Source: CAD feature listing. Evaluate the final solid. Frame: model axes, mm. A direction names the side the tool comes from. Give positions to 0.01 mm unless a question says otherwise; leave off trailing zeros. Order: outer loops, then holes, each group sorted by start corner. A loop starts at its lowest first (then second) coordinate and runs counter-clockwise, first axis right, second up.
1) Access query for faces 4 (the face through (-3, 1.27, -55)), 5 (the face through (-5.3, 4.3, 0)). Directions: +Z, -Z, +X, -X, +Y, -Y. A direction counts if a zero-diameter tool reaches every point of the face in a straight line with its end or side. Return the directions, or none.
2) Section B-B, the plane z = -102. Return loops of the section in (x, y), plus the area to 3 significant figures.
3) First-contact query: P1, Ø2, axis at y = 8, z = -45.5, coming from the -X side; P2, Ø4, axis at y = 6.5, z = -90.5, coming from the -X side; P3, Ø1.7, axis at y = 3, z = -53.5, coming from the +X side. Flat tips, straight axial feed; report the tip coordinate or a pass-through.
4) Draft query along Y for faces 1 (the face through (-5.08, 3, -55)), 2 (the face through (-3, 0, -55)), 3 (the face through (-5.3, 4.3, -111.125)). Return one class per face: released by +Y, released by -Y, zero draft, split by the parting line, or undercut.
5) Section C-C, the plane y = 8.5. Return loops of the section in (x, z) (3 decimals).
6) Section A-A, the plane x = -1. Return loops of the section in (y, z) (3 decimals), plus the area to 3 significant figures.
7) Material intervals for line 1 (Y direction, x = -0.25, z = -51); line 2 (X direction, y = 4.25, z = -14.5); line 3 (Y direction, x = -3, z = -29.5), sorted ascending.
```python
from build123d import *

# Parameters (mm, degrees)
EXTRUDE_THIN1_DEPTH = 111.125
FILLET1_R           = 1.27


with BuildPart() as part:
    # Sketch1 → Extrude-Thin1 (new body)
    with BuildSketch(Plane.XY):
        with BuildLine():
            Line((0, 0), (-6.35, 0))
            Line((-6.35, 0), (-6.35, 4.7625))
            ThreePointArc((-6.35, 4.7625), (-4.490128061, 9.252628061), (0, 11.1125))
            Line((0, 11.1125), (0, 9.8425))
            ThreePointArc((0, 9.8425), (-3.592102448, 8.354602448), (-5.08, 4.7625))
            Line((-5.08, 4.7625), (-5.08, 1.27))
            Line((-5.08, 1.27), (0, 1.27))
            Line((0, 1.27), (0, 0))
        make_face()
    extrude(amount=-EXTRUDE_THIN1_DEPTH)

    # Fillet1
    fillet1_edges = [part.edges().sort_by_distance(p)[0] for p in [
        (-6.35, 0, -55.5625),
    ]]
    fillet(fillet1_edges, radius=FILLET1_R)


solid = part.part
```
From the geometry:
1. face 4: +Z, -Z, +X
1. face 5: +Z, +X, -X, +Y, -Y
2. outline: (-6.35, 1.27) arc R1.27 ccw to (-5.08, 0) - (0, 0) - (0, 1.27) - (-5.08, 1.27) - (-5.08, 4.76) arc R5.08 cw to (0, 9.84) - (0, 11.11) arc R6.35 ccw to (-6.35, 4.76) - close
2. area: 23.6 mm2
3. P1: stops at x = -5.94
3. P2: stops at x = -6.35
3. P3: stops at x = -5.08
4. face 1: undercut
4. face 2: released by -Y
4. face 3: zero draft
5. outline: (-5.134, -111.125) - (-3.441, -111.125) - (-3.441, 0) - (-5.134, 0) - close
6. outline: (0, -111.125) - (1.27, -111.125) - (1.27, 0) - (0, 0) - close; (9.743, -111.125) - (11.033, -111.125) - (11.033, 0) - (9.743, 0) - close
6. area: 284 mm2
7. line 1: y = 0 to 1.27, 9.84 to 11.11
7. line 2: x = -6.35 to -5.08
7. line 3: y = 0 to 1.27, 8.86 to 10.36
